from build123d import *

# Parameters (mm, degrees)
F0_R        = 11
F0_R_2      = 4.5
F1_DEPTH    = 18
F2_DEPTH    = 10
F3_T1_DEPTH = 66.9897948557


# Not quite as in the source:
# - a fillet or chamfer that OpenCascade refuses, or shapes differently, is made with other operations: its cross-section is extruded or revolved along the edge and cut away or added
# - a feature names something its author has since deleted; it is built from what else it names


with BuildPart() as f1:
    # F0 (on Front) → F1 (new body)
    with BuildSketch(Plane.XZ):
        with BuildLine():
            Line((-47.1908605099, -35.0622619203), (-327.1908605099, -35.0622619203))
            Line((-327.1908605099, -35.0622619203), (-327.1908605099, -58.0622619203))
            Line((-327.1908605099, -58.0622619203), (-292.1908605099, -58.0622619203))
            ThreePointArc((-292.1908605099, -58.0622619203), (-287.1908605099, -53.0622619203), (-282.1908605099, -58.0622619203))
            ThreePointArc((-282.1908605099, -58.0622619203), (-284.9547925324, -62.5343978753), (-290.1908605099, -62.0622619203))
            Line((-290.1908605099, -62.0622619203), (-327.1908605099, -62.0622619203))
            Line((-327.1908605099, -62.0622619203), (-327.1908605099, -70.0622619203))
            Line((-327.1908605099, -70.0622619203), (-47.1908605099, -70.0622619203))
            Line((-47.1908605099, -70.0622619203), (-47.1908605099, -62.0622619203))
            Line((-47.1908605099, -62.0622619203), (-84.1908605099, -62.0622619203))
            ThreePointArc((-84.1908605099, -62.0622619203), (-91.6629964649, -55.8261939428), (-82.1908605099, -58.0622619203))
            Line((-82.1908605099, -58.0622619203), (-47.1908605099, -58.0622619203))
            Line((-47.1908605099, -58.0622619203), (-47.1908605099, -35.0622619203))
        make_face()
        with Locations((-187.1908605099, -58.0622619203)):
            Circle(F0_R, mode=Mode.SUBTRACT)
        with Locations((-187.1908605099, -58.0622619203)):
            Circle(F0_R)
        with Locations((-187.1908605099, -58.0622619203)):
            Circle(F0_R_2, mode=Mode.SUBTRACT)
    extrude(amount=F1_DEPTH)

    # F0 (on Front) → F2 (cut)
    with BuildSketch(Plane.XZ):
        with Locations((-187.1908605099, -58.0622619203)):
            Circle(F0_R)
        with Locations((-187.1908605099, -58.0622619203)):
            Circle(F0_R_2, mode=Mode.SUBTRACT)
    extrude(amount=F2_DEPTH, mode=Mode.SUBTRACT)

    # F3: fillet of radius 10 on 2 edges, made by hand

    # F3_s2 → F3_t1 (cut)
    with BuildSketch(Plane.XZ.offset(-24.4948974278)):
        with BuildLine():
            ThreePointArc((-317.3929015387, -70.0622619203), (-323.7174568591, -67.8082286127), (-327.1908605099, -62.0622619203))
            Line((-327.1908605099, -62.0622619203), (-327.1908605099, -70.0622619203))
            Line((-327.1908605099, -70.0622619203), (-317.3929015387, -70.0622619203))
        make_face()
        with BuildLine():
            ThreePointArc((-47.1908605099, -62.0622619203), (-50.6642641607, -67.8082286127), (-56.988819481, -70.0622619203))
            Line((-56.988819481, -70.0622619203), (-47.1908605099, -70.0622619203))
            Line((-47.1908605099, -70.0622619203), (-47.1908605099, -62.0622619203))
        make_face()
    extrude(amount=F3_T1_DEPTH, mode=Mode.SUBTRACT)


solid = f1.part
Check sheet for the modelled part. Datum: model origin and axes. Units: mm. A direction names the side the tool comes from. Round coordinates to 2 decimals unless told otherwise and drop trailing zeros. Write each loop counter-clockwise with the first axis right and the second up, starting at its lowest first coordinate (ties: lowest second). Pieces come first, ordered by that corner, then holes. Notation, with made-up numbers: (-16, 7.5) - (36, 7.5) arc R17 cw to (36, 39.5) - close; hole circle Ø4 at (81, -11). An arc over 180 degrees is marked (long way). Return JSON: item names as keys, results as strings.
Q1. Draft check along X on faces 4 (the cylindrical face through (-185.11, -13.94, -62.05)), 5 (the flat face through (-310, -9, -58.062)), 6 (the cylindrical face through (-282.806, -8.874, -55.66)), 7 (the flat face through (-47.191, -9, -47)). Enter one of: released by +X, released by -X, zero draft, split by the parting line, or undercut.
Returned:
{"face 4": "undercut", "face 5": "zero draft", "face 6": "undercut", "face 7": "released by +X"}
Q2. Scan lines: L1, parallel to X at y = -16.75, z = -55; L2, parallel to Z at x = -310.5, y = -15.75; L3, parallel to X at y = -12.25, z = -57 (3 decimals). Record each from-to range of solid material in increasing order. Write a range as from..to.
Returned:
{"L1": "x = -327.19..-291.14, -283.24..-190.49, -183.89..-91.14, -83.24..-47.19", "L2": "z = -70.06..-62.06, -58.06..-35.06", "L3": "x = -327.191..-292.077, -282.305..-191.564, -182.818..-92.077, -82.305..-47.191"}
Q3. Cross-section at C-C (y = -3.25). Record the boundary of the cut face in (x, z), then the cut area to 3 significant figures.
Returned:
{"outline": "(-327.19, -62.06) arc R10 ccw to (-317.39, -70.06) - (-56.99, -70.06) arc R10 ccw to (-47.19, -62.06) - (-84.19, -62.06) arc R5 cw (long way) to (-82.19, -58.06) - (-47.19, -58.06) - (-47.19, -35.06) - (-327.19, -35.06) - (-327.19, -58.06) - (-292.19, -58.06) arc R5 cw (long way) to (-290.19, -62.06) - close; hole circle Ø22 at (-187.19, -58.06)", "area": "8,940 mm²"}
Q4. Cross-section at B-B (x = -67.5). Record the boundary of the cut face in (y, z), then the cut area to 3 significant figures.
Returned:
{"outline": "(-18, -70.06) - (0, -70.06) - (0, -62.06) - (-18, -62.06) - close; (-18, -58.06) - (0, -58.06) - (0, -35.06) - (-18, -35.06) - close", "area": "558 mm²"}
Q5. Cross-section at D-D (z = -66). Record the boundary of the cut face in (x, y), then the cut area to 3 significant figures.
Returned:
{"outline": "(-325.44, -18) - (-48.94, -18) - (-48.94, 0) - (-179.58, 0) - (-179.58, -10) - (-194.81, -10) - (-194.81, 0) - (-325.44, 0) - close", "area": "4,820 mm²"}
Q6. Access from +Z, -Z, +X, -X, +Y, -Y to the whole of each face (thin tool, end or side, straight path). Record for faces 1 (the cylindrical face through (-195.3, -4.93, -50.63)), 2 (the flat face through (-308, -9, -62.062)), 3 (the flat face through (-65, -9, -62.062)).
Returned:
{"face 1": "+Y", "face 2": "-X, +Y, -Y", "face 3": "+X, +Y, -Y"}
Q7. Cross-section at A-A (y = -15.5). Record the boundary of the cut face in (x, z).
Returned:
{"outline": "(-327.19, -62.06) arc R10 ccw to (-317.39, -70.06) - (-56.99, -70.06) arc R10 ccw to (-47.19, -62.06) - (-84.19, -62.06) arc R5 cw (long way) to (-82.19, -58.06) - (-47.19, -58.06) - (-47.19, -35.06) - (-327.19, -35.06) - (-327.19, -58.06) - (-292.19, -58.06) arc R5 cw (long way) to (-290.19, -62.06) - close; hole circle Ø9 at (-187.19, -58.06)"}
Q8. Depth check by flat-ended pin: P1, Ø4, axis at x = -189, z = -64.5, coming from the +Y side; P2, Ø9, axis at x = -287.19, z = -58.06, coming from the -Y side. Enter the tip coordinate at first touch or a pass-through.
Returned:
{"P1": "stops at y = -10", "P2": "passes through"}
